Part model, mm, in its own coordinate system. A direction names the side the tool comes from. Coordinates: 2 decimals unless noted, no trailing zeros. Loops run counter-clockwise (first coordinate to the right, second up) from the corner with the lowest first, then second, coordinate; pieces in that order, holes last. Notation, with made-up numbers: (49.5, -32) - (57.5, -32) arc R20 ccw to (57.5, -10) - close; hole circle Ø7 at (-2, 30.5). An arc over 180 degrees is marked (long way). Use a Markdown table: item, result. Add a question column.
1) Band-saw the part on B-B (y = 124). Give the cut face in (x, z), plus the area to 3 significant figures.
2) Band-saw the part on A-A (y = 165). Give the cut face in (x, z), plus the area to 3 significant figures.
3) Tool access for faces 4 (the face through (3, 121, -22)), 5 (the face through (0, 121, -20)), 6 (the face through (1.6, 195.1, -5.5)): list every direction of +Z, -Z, +X, -X, +Y, -Y with a clear straight run to the whole face (end or side of a thin tool).
4) Probe probe 1 along X at (y, z) = (231, -28); probe 2 along Z at (x, y) = (29, 156); probe 3 along X at (y, z) = (48.5, -5). List the from-to ranges inside material, lowest first. Write a range as [from, to].
5) Drop flat-ended pins along their axis: P1, Ø6, axis at x = 33, y = 151, coming from the -Z side; P2, Ø15, axis at y = 122.5, z = -28.5, coming from the +X side; P3, Ø0.9, axis at x = 2, z = -14.5, coming from the -Y side; P4, Ø12, axis at x = 10, y = 112.5, coming from the -Z side. Give the stop position or say it passes through.
6) Band-saw the part on C-C (x = 29). Give the cut face in (y, z), plus the area to 3 significant figures.
7) Pull direction Y, two halves, no side cores. Call faces 1 (the face through (1.6, 165.1, -5.5)), 2 (the face through (11, 0, -2)), 3 (the face through (11, 245, -2)): +Y half, -Y half, draft (parallel to the pull), parting line (faces both ways), or undercut.
from build123d import *

# Parameters (mm, degrees)
IRON_V40X40X3_1_DEPTH = 245
CUT_EXTRUDE1_DEPTH    = 10


with BuildPart() as part:
    # Sketch1 → Iron V40X40X3(1) (new body)
    with BuildSketch(Plane(origin=(0, 0, 0), x_dir=(1, 0, 0), z_dir=(0, 1, 0))):
        with BuildLine():
            Line((0, 0), (0, 40))
            ThreePointArc((0, 40), (2.121320344, 39.121320344), (3, 37))
            Line((3, 37), (3, 6.5))
            ThreePointArc((3, 6.5), (4.025126266, 4.025126266), (6.5, 3))
            Line((6.5, 3), (37, 3))
            ThreePointArc((37, 3), (39.121320344, 2.121320344), (40, 0))
            Line((40, 0), (0, 0))
        make_face()
    extrude(amount=IRON_V40X40X3_1_DEPTH)

    # Sketch2 → Cut-Extrude1 (cut)
    with BuildSketch(Plane.ZY):
        with BuildLine():
            Line((-25.5, 170), (-10.5, 170))
            ThreePointArc((-10.5, 170), (-5.5, 165), (-10.5, 160))
            Line((-10.5, 160), (-25.5, 160))
            ThreePointArc((-25.5, 160), (-30.5, 165), (-25.5, 170))
        make_face()
        with BuildLine():
            Line((-25.5, 200), (-10.5, 200))
            ThreePointArc((-10.5, 200), (-5.5, 195), (-10.5, 190))
            Line((-10.5, 190), (-25.5, 190))
            ThreePointArc((-25.5, 190), (-30.5, 195), (-25.5, 200))
        make_face()
    extrude(amount=-CUT_EXTRUDE1_DEPTH, mode=Mode.SUBTRACT)


solid = part.part
Answer block:
| question | item | result |
|---|---|---|
| 1 | outline | (0, -40) arc R3 ccw to (3, -37) - (3, -6.5) arc R3.5 cw to (6.5, -3) - (37, -3) arc R3 ccw to (40, 0) - (0, 0) - close |
| 1 | area | 230 mm2 |
| 2 | outline | (0, -40) arc R3 ccw to (3, -37) - (3, -30.5) - (0, -30.5) - close; (0, -5.5) - (3.15, -5.5) arc R3.5 cw to (6.5, -3) - (37, -3) arc R3 ccw to (40, 0) - (0, 0) - close |
| 2 | area | 155 mm2 |
| 3 | face 4 | -Z, +X, +Y, -Y |
| 3 | face 5 | +Z, -Z, -X, +Y, -Y |
| 3 | face 6 | +X, -X |
| 4 | probe 1 | [0, 3] |
| 4 | probe 2 | [-3, 0] |
| 4 | probe 3 | [0, 3.34] |
| 5 | P1 | z = -3 |
| 5 | P2 | x = 3 |
| 5 | P3 | y = 0 |
| 5 | P4 | z = -4.05 |
| 6 | outline | (0, -3) - (245, -3) - (245, 0) - (0, 0) - close |
| 6 | area | 735 mm2 |
| 7 | face 1 | undercut |
| 7 | face 2 | -Y half |
| 7 | face 3 | +Y half |
